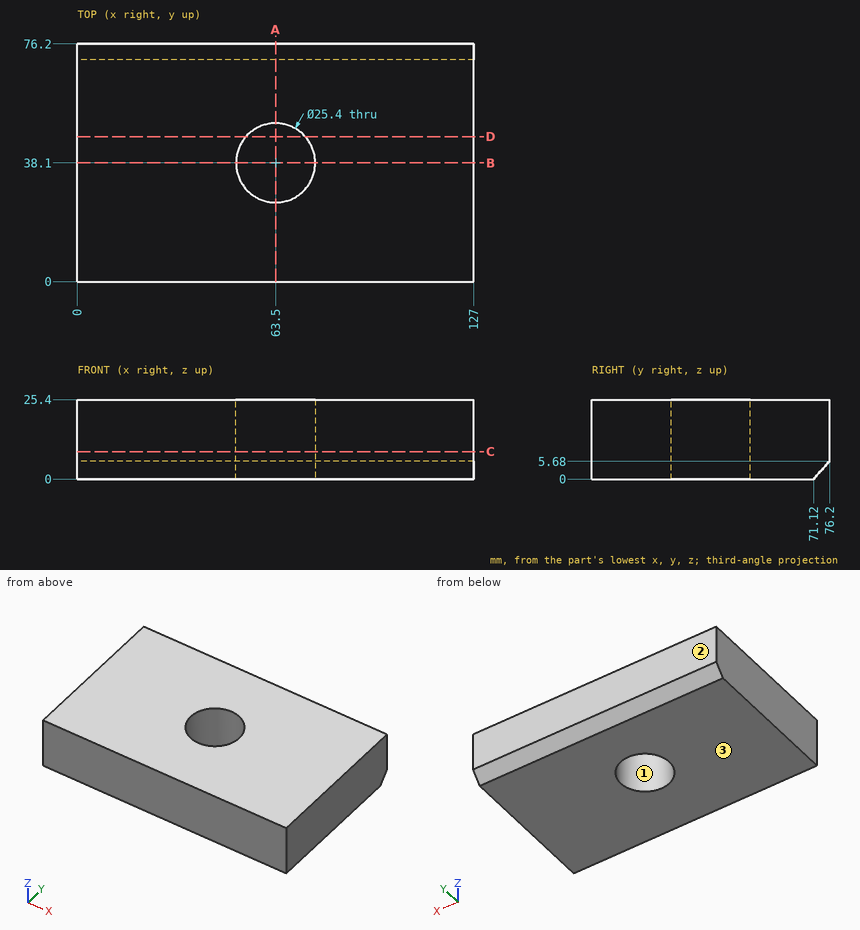
Geometry check sheet. Reference: drawing and pictorial views, mm from the part's lowest x, y, z. Give positions to 0.01 mm unless a question says otherwise; leave off trailing zeros. Write each loop counter-clockwise with the first axis right and the second up, starting at its lowest first coordinate (ties: lowest second). Pieces come first, ordered by that corner, then holes. Notation, with made-up numbers: (40, -11) - (99, -11) arc R20 cw to (99, 16) - close; hole circle Ø8 at (-16.75, -28). An arc over 180 degrees is marked (long way). Use a Markdown table: item, result.
Q1. Section check A-A, the plane x = 63.5. Enter the section's corners in (y, z), then the cut area to 3 significant figures.
Computed:
| item | result |
|---|---|
| outline | (0, 0) - (25.4, 0) - (25.4, 25.4) - (0, 25.4) - close; (50.8, 0) - (71.12, 0) - (76.2, 5.68) - (76.2, 25.4) - (50.8, 25.4) - close |
| area | 1,280 mm² |
Q2. Section check B-B, the plane y = 38.1. Enter the section's corners in (x, z).
Computed:
| item | result |
|---|---|
| outline | (0, 0) - (50.8, 0) - (50.8, 25.4) - (0, 25.4) - close; (76.2, 0) - (127, 0) - (127, 25.4) - (76.2, 25.4) - close |
Q3. Section check C-C, the plane z = 8.75. Enter the section's corners in (x, y).
Computed:
| item | result |
|---|---|
| outline | (0, 0) - (127, 0) - (127, 76.2) - (0, 76.2) - close; hole circle Ø25.4 at (63.5, 38.1) |
Q4. Go/stop test with a flat-tipped pin: P1, Ø15, axis at x = 63.5, y = 38.1, coming from the +Z side. Record where the tip stops, or that it passes through.
Computed:
| item | result |
|---|---|
| P1 | passes through |
Q5. Draft check along Y on the marked faces 1, 2 and 3. Enter one of: pulls with the +Y half, pulls with the -Y half, needs draft (parallel to the pull), parting line crosses it, or undercut.
Computed:
| item | result |
|---|---|
| face 1 | undercut |
| face 2 | pulls with the +Y half |
| face 3 | needs draft |
Q6. Section check D-D, the plane y = 46.5. Enter the section's corners in (x, z) (1 decimal).
Computed:
| item | result |
|---|---|
| outline | (0, 0) - (54, 0) - (54, 25.4) - (0, 25.4) - close; (73, 0) - (127, 0) - (127, 25.4) - (73, 25.4) - close |
Q7. Thickness scan on L1, parallel to Y at x = 63.5, z = 9; L2, parallel to Y at x = 57.5, z = 8; L3, parallel to X at y = 42.5, z = 18.75. Record the ranges inside material, lowest first. Write a range as [from, to].
Computed:
| item | result |
|---|---|
| L1 | y = [0, 25.4], [50.8, 76.2] |
| L2 | y = [0, 26.91], [49.29, 76.2] |
| L3 | x = [0, 51.59], [75.41, 127] |
